```python
from build123d import *

# Parameters (mm, degrees)
F0_R      = 25.4
F1_DEPTH  = 152.4
F3_DEPTH  = 38.1
F4_R      = 31.75
F5_DEPTH  = 38.1
F6_R      = 88.9
F7_DEPTH  = 38.1
F9_R      = 12.7
F10_DEPTH = 152.401


with BuildPart() as f1:
    # F0 (on Top) → F1 (new body)
    with BuildSketch(Plane.XY):
        Circle(F0_R)
    extrude(amount=-F1_DEPTH)

    # F2 (on Right) → F3 (join, symmetric)
    with BuildSketch(Plane.YZ):
        Polygon((50.8, 25.4), (0, 25.4), (-50.8, 25.4), (-50.8, 88.9), (-76.2, 88.9), (-76.2, 0), (0, 0), (76.2, 0), (76.2, 88.9), (50.8, 88.9), align=None)
    extrude(amount=F3_DEPTH, both=True)

    # F4 (on Front) → F5 (join, symmetric)
    with BuildSketch(Plane.XZ):
        with Locations((0, -152.4)):
            Circle(F4_R)
    extrude(amount=F5_DEPTH, both=True)

    # F6 (on face) → F7 (join)
    with BuildSketch(Plane.XZ.offset(38.1)):
        with Locations((0, -152.4)):
            Circle(F6_R)
    extrude(amount=F7_DEPTH)

    # F8: F1 across plane


with BuildPart() as f1_1:
    add(f1.part)
    add(f1.part.mirror(Plane.XZ))

    # F9 (on face) → F10 (cut, through all)
    with BuildSketch(Plane.XZ.offset(76.2)):
        with Locations((0, 63.5)):
            Circle(F9_R)
    extrude(amount=-F10_DEPTH, mode=Mode.SUBTRACT)


solid = f1_1.part
```
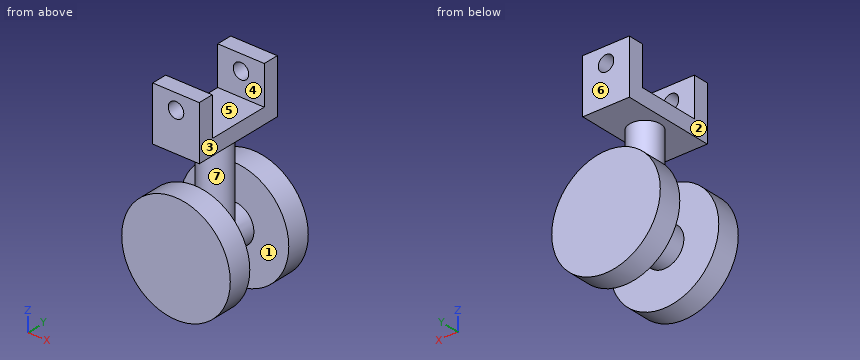
The model under review builds one solid part; all positions refer to its coordinate system, in mm. Face numbers are marked on the shaded views. A direction names the side the tool comes from. Give positions to 0.01 mm unless a question says otherwise; leave off trailing zeros. Write each loop counter-clockwise with the first axis right and the second up, starting at its lowest first coordinate (ties: lowest second). Pieces come first, ordered by that corner, then holes.
(1) The part is to be moulded in two halves that separate along Z. For the marked faces 5, 6 and 7, say which applies: released by +Z, released by -Z, zero draft, split by the parting line, or undercut.
(2) Consider section A-A, the plane y = 62. Give the boundary of the cut face in (x, z), and give its area (3 significant figures).
(3) For P1, Ø3, axis at y = 15, z = -65.5, coming from the -X side; P2, Ø12, axis at x = -22, y = 4.5, coming from the -Z side; P3, Ø6, axis at x = -68.5, y = -57.5, coming from the -Z side, all flat-tipped, find the tip position at first contact; note any pin that passes through.
(4) To check wall thickness, follow L1, parallel to Z at x = 0, y = -68.5; L2, parallel to X at y = 68, z = 63; L3, parallel to Y at x = -34, z = -184.5. State the ranges of each line that lie inside material, in increasing order.
(5) Consider section C-C, the plane x = 0. Give the number of separate pieces and of enclosed holes in the cut face, and give its area (3 significant figures).
(6) Consider section B-B, the plane z = 63.5. Give the boundary of the cut face in (x, y), and give its area (3 significant figures).
(7) Consider section D-D, the plane x = 48.5. Give the boundary of the cut face in (y, z).
(8) Tool access review of the marked faces 1, 2, 3 and 4: name each direction out of +Z, -Z, +X, -X, +Y, -Y from which nothing blocks a thin tool from reaching the whole face with its end or side.
Returned:
1. face 5: released by +Z
1. face 6: zero draft
1. face 7: undercut
2. outline: circle Ø177.8 at (0, -152.4); (-38.1, 0) - (38.1, 0) - (38.1, 88.9) - (-38.1, 88.9) - close; hole circle Ø25.4 at (0, 63.5)
2. area: 31,100 mm2
3. P1: stops at x = -21.52
3. P2: stops at z = -179.82
3. P3: stops at z = -212.51
4. L1: z = -241.3 to -63.5, 0 to 50.8, 76.2 to 88.9
4. L2: x = -38.1 to -12.69, 12.69 to 38.1
4. L3: y = -76.2 to -38.1, 38.1 to 76.2
5. separate pieces: 3
5. enclosed holes: 0
5. area: 30,300 mm2
6. outline: (-38.1, -76.2) - (-12.7, -76.2) - (-12.7, -50.8) - (-38.1, -50.8) - close; (-38.1, 50.8) - (-12.7, 50.8) - (-12.7, 76.2) - (-38.1, 76.2) - close; (12.7, -76.2) - (38.1, -76.2) - (38.1, -50.8) - (12.7, -50.8) - close; (12.7, 50.8) - (38.1, 50.8) - (38.1, 76.2) - (12.7, 76.2) - close
6. area: 2,580 mm2
7. outline: (-76.2, -226.9) - (-38.1, -226.9) - (-38.1, -77.9) - (-76.2, -77.9) - close; (38.1, -226.9) - (76.2, -226.9) - (76.2, -77.9) - (38.1, -77.9) - close
8. face 1: none
8. face 2: +Z, -X, +Y, -Y
8. face 3: +Z, +X, +Y, -Y
8. face 4: +Z, +X, -X
